Answer from the drawing. Dimensions are ordinates in mm from the lowest x, y and z of the part. A direction names the side the tool comes from. Coordinates: 2 decimals unless noted, no trailing zeros. Write each loop counter-clockwise with the first axis right and the second up, starting at its lowest first coordinate (ties: lowest second). Pieces come first, ordered by that corner, then holes. Notation, with made-up numbers: M 50,19 L 99,19 A25 cw 99,56 Z; hole C 75.5,49 d5. An arc over 180 degrees is marked long. Put each result on its own line as item: value. Start each with the question number.
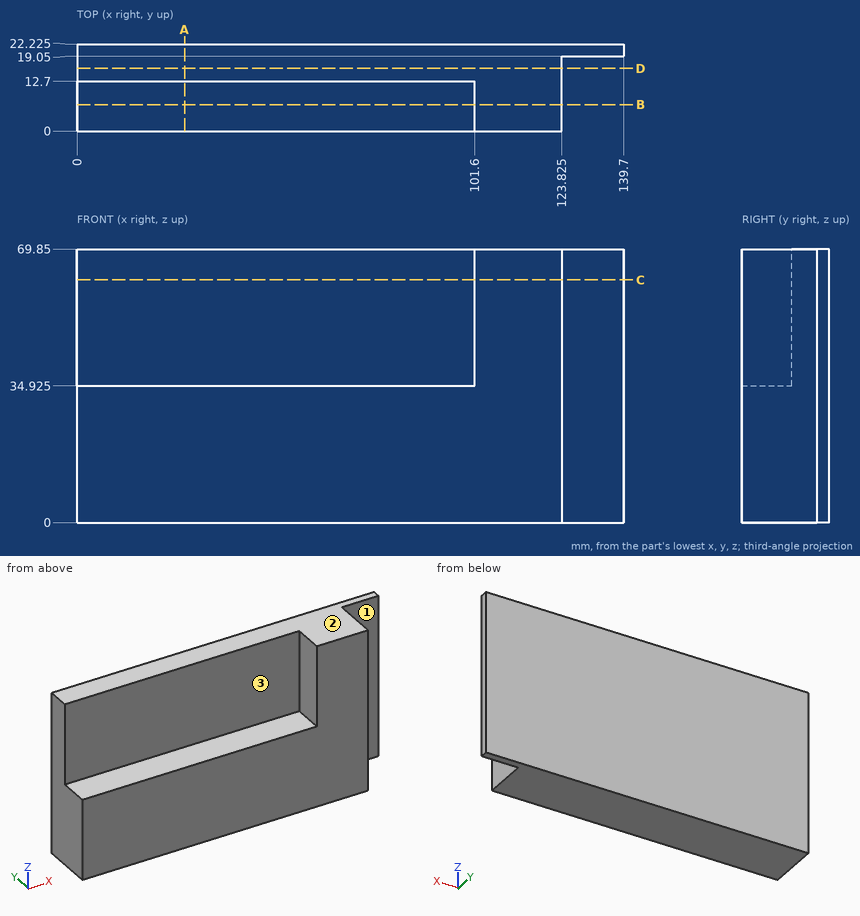
1) Given pin 1 Ø6.5 at (y, z) = (9, 46.5) entering from -X; pin 2 Ø8 at (x, z) = (50.5, 56) entering from -Y; pin 3 Ø5.5 at (y, z) = (12, 34.5) entering from +X (3 decimals), each flat-ended and moving along its own axis, determine where each tip first touches the part or whether it passes through.
2) Straight lines are drawn through the part: probe 1 along X at (y, z) = (1.5, 47) (3 decimals); probe 2 along Y at (x, z) = (89, 53.5) (3 decimals); probe 3 along X at (y, z) = (18, 19.5) (3 decimals). For each, find the intervals that lie inside material, in ascending order.
3) For the marked faces 1, 2 and 3, determine the directions among +Z, -Z, +X, -X, +Y, -Y from which every point of the face is accessible in a straight line to the end or side of a thin tool.
4) A cutting plane is placed at C-C on z = 62. Write down the section's boundary in (x, y) (3 decimals), then the cut area to 3 significant figures.
5) A cutting plane is placed at D-D on y = 16. Write down the section's boundary in (x, z) (3 decimals), then the cut area to 3 significant figures.
6) A cutting plane is placed at A-A on x = 27.5. Write down the section's boundary in (y, z) (3 decimals), then the cut area to 3 significant figures.
7) A cutting plane is placed at B-B on y = 6.75. Write down the section's boundary in (x, z) (3 decimals), then the cut area to 3 significant figures.
Answers follow:
1. pin 1: stops at x = 101.6
1. pin 2: stops at y = 12.7
1. pin 3: stops at x = 123.825
2. probe 1: x = 101.6 to 123.825
2. probe 2: y = 12.7 to 22.225
2. probe 3: x = 0 to 123.825
3. face 1: +Z, -Z, +X, -Y
3. face 2: +Z, +X, -X, +Y, -Y
3. face 3: +Z, -X, -Y
4. outline: M 0,12.7 L 101.6,12.7 L 101.6,0 L 123.825,0 L 123.825,19.05 L 139.7,19.05 L 139.7,22.225 L 0,22.225 Z
4. area: 1,510 mm²
5. outline: M 0,0 L 123.825,0 L 123.825,69.85 L 0,69.85 Z
5. area: 8,650 mm²
6. outline: M 0,0 L 22.225,0 L 22.225,69.85 L 12.7,69.85 L 12.7,34.925 L 0,34.925 Z
6. area: 1,110 mm²
7. outline: M 0,0 L 123.825,0 L 123.825,69.85 L 101.6,69.85 L 101.6,34.925 L 0,34.925 Z
7. area: 5,100 mm²
